Print and shaded views of the part. All mm, measured from the part's lowest x, y and z. Round coordinates to 2 decimals unless told otherwise and drop trailing zeros. Write each loop counter-clockwise with the first axis right and the second up, starting at its lowest first coordinate (ties: lowest second). Pieces come first, ordered by that corner, then holes. Notation, with made-up numbers: (-21.5, 54) - (7.5, 54) arc R29 ccw to (7.5, 87) - close; hole circle Ø8 at (80.25, 39.5). An arc over 180 degrees is marked (long way). Put each result on its own line as item: value. Start each with the question number.
Item 1: Cut at A-A (z = 0.9). Give the cut face in (x, y).
Item 2: Drill centre lines: line 1 (Y direction, x = 2.54, z = 0.65); line 2 (X direction, y = 3, z = 0.9); line 3 (X direction, y = 3.5, z = 0.25). Where is each one in solid material? Low to high. Write a range as from..to.
Item 3: Cut at B-B (y = 2.25). Give the cut face in (x, z), and give its area (3 significant figures).
Item 4: Pin check, flat tips, straight feed: pin 1 Ø1.5 at (x, y) = (27.94, 15.494) entering from -Z; pin 2 Ø4 at (x, y) = (27.94, 2.54) entering from +Z. Stop position of each tip, or through.
Item 5: Cut at C-C (x = 3.5). Give the cut face in (y, z), and give its area (3 significant figures).
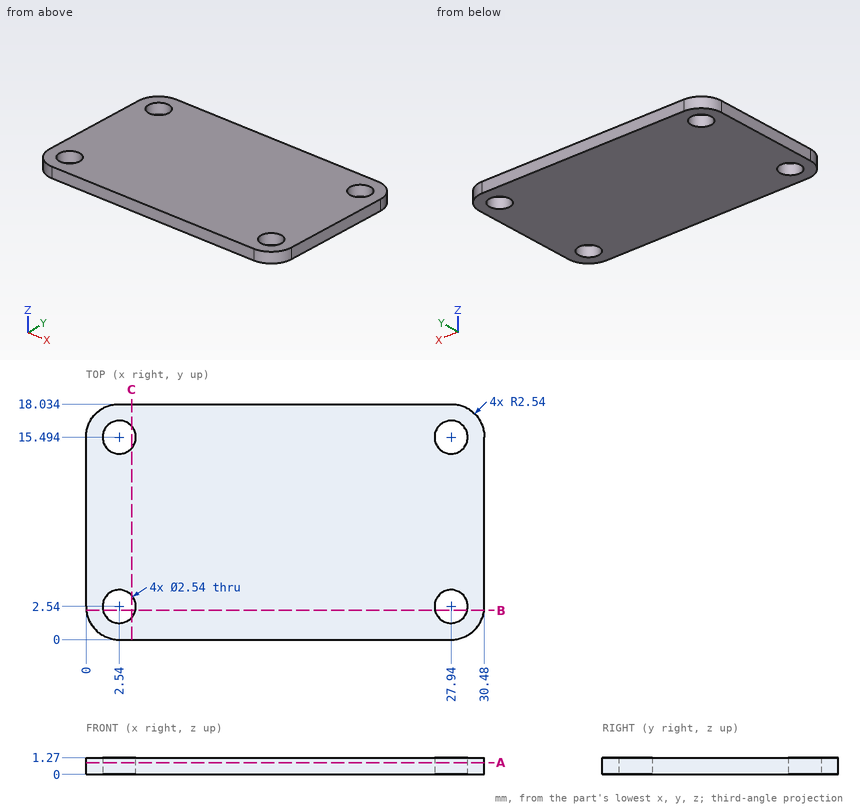
Output values:
1. outline: (0, 2.54) arc R2.54 ccw to (2.54, 0) - (27.94, 0) arc R2.54 ccw to (30.48, 2.54) - (30.48, 15.49) arc R2.54 ccw to (27.94, 18.03) - (2.54, 18.03) arc R2.54 ccw to (0, 15.49) - close; hole circle Ø2.54 at (2.54, 2.54); hole circle Ø2.54 at (2.54, 15.49); hole circle Ø2.54 at (27.94, 2.54); hole circle Ø2.54 at (27.94, 15.49)
2. line 1: 0..1.27, 3.81..14.22, 16.76..18.03
2. line 2: 0..1.36, 3.72..26.76, 29.12..30.48
2. line 3: 0..1.71, 3.37..27.11, 28.77..30.48
3. outline: (0.02, 0) - (1.3, 0) - (1.3, 1.27) - (0.02, 1.27) - close; (3.78, 0) - (26.7, 0) - (26.7, 1.27) - (3.78, 1.27) - close; (29.18, 0) - (30.46, 0) - (30.46, 1.27) - (29.18, 1.27) - close
3. area: 32.4 mm2
4. pin 1: through
4. pin 2: z = 1.27
5. outline: (0, 0) - (1.71, 0) - (1.71, 1.27) - (0, 1.27) - close; (3.37, 0) - (14.66, 0) - (14.66, 1.27) - (3.37, 1.27) - close; (16.33, 0) - (18.03, 0) - (18.03, 1.27) - (16.33, 1.27) - close
5. area: 18.7 mm2
